Input: part model. Units: mm. Frame: model coordinates. A direction names the side the tool comes from. Round coordinates to 2 decimals unless told otherwise and drop trailing zeros. Loops run counter-clockwise (first coordinate to the right, second up) from the corner with the lowest first, then second, coordinate; pieces in that order, holes last. Notation, with made-up numbers: (11.5, 44.25) - (55.5, 44.25) arc R16 ccw to (55.5, 53.25) - close; hole circle Ø11 at (62, -23.75). An arc over 180 degrees is marked (long way). Write each question's results on one line, items separated by ' | '.
from build123d import *

# Parameters (mm, degrees)
F1_DEPTH = 25
F2_R     = 0.8


# Not quite as in the source:
# - a feature names something its author has since deleted; it is built from what else it names


with BuildPart() as f1:
    # F0 (on Top) → F1 (new body)
    with BuildSketch(Plane.XY):
        Polygon((-15.2705168036, 4.776119403), (-17.6585765051, -2.8591389988), (-14.7953546044, -3.7546613869), (-13.302817291, 1.0173751143), (-3.7587442887, -1.9676995126), (-21.9676995126, -60.1865448263), (-31.5117725148, -57.2014701994), (-30.0192352014, -52.4294336983), (-32.8824571021, -51.5339113102), (-35.2705168036, -59.169169712), (-20, -63.945289115), (-19.0616978853, -60.945289115), (-0.4691510573, -1.5), (3.1308489427, -1.5), (3.1308489427, -10), (6.1308489427, -10), (6.1308489427, -4.0311980993), (6.1308489427, 0), (0, 0), align=None)
        Polygon((0, -60.945289115), (-19.0616978853, -60.945289115), (-20, -63.945289115), (0, -63.945289115), align=None)
        Polygon((9.5918557882, -1.385692507), (6.1308489427, 0), (6.1308489427, -4.0311980993), (9.5918557882, -2.7201510966), align=None)
    extrude(amount=F1_DEPTH)

    # F2
    f2_edges = [f1.edges().sort_by_distance(p)[0] for p in [
        (-15.270517, 4.776119, 12.5),
        (-17.658577, -2.859139, 12.5),
        (-14.795355, -3.754661, 12.5),
        (-32.882457, -51.533911, 12.5),
        (-35.270517, -59.16917, 12.5),
        (-30.019235, -52.429434, 12.5),
        (-20, -63.945289, 12.5),
        (6.130849, -10, 12.5),
        (3.130849, -10, 12.5),
        (0, -60.945289, 12.5),
        (0, -63.945289, 12.5),
        (9.591856, -1.385693, 12.5),
        (9.591856, -2.720151, 12.5),
        (0, 0, 12.5),
        (6.130849, 0, 12.5),
        (6.130849, -4.031198, 12.5),
    ]]
    fillet(f2_edges, radius=F2_R)


solid = f1.part
1. Section query A-A, the plane x = -1.5. Output: boundary loops of the cut face in (y, z).
Answer:
outline: (-63.95, 0) - (-60.95, 0) - (-60.95, 25) - (-63.95, 25) - close; (-4.8, 0) - (0.47, 0) - (0.47, 25) - (-4.8, 25) - close
2. Section query C-C, the plane y = -30.5. Output: boundary loops of the cut face in (x, z).
Answer:
outline: (-12.68, 0) - (-9.54, 0) - (-9.54, 25) - (-12.68, 25) - close
3. Section query B-B, the plane x = -10. Output: boundary loops of the cut face in (y, z), plus the area to 3 significant figures.
Answer:
outline: (-63.95, 0) - (-60.95, 0) - (-60.95, 25) - (-63.95, 25) - close; (-31.97, 0) - (-21.92, 0) - (-21.92, 25) - (-31.97, 25) - close; (-0.02, 0) - (3.13, 0) - (3.13, 25) - (-0.02, 25) - close | area: 405 mm^2
4. Contact query for flat-ended pins moving along their axis: pin 1 (8 mm diameter, centred on x = 4.5, z = 20, fed in from +Y); pin 2 (10 mm diameter, centred on y = -12.5, z = 7.5, fed in from -X); pin 3 (1.4 mm diameter, centred on y = -7.5, z = 14, fed in from +X). Output: stop coordinate, or through.
Answer:
pin 1: y = 0 | pin 2: x = -8.62 | pin 3: x = 6.13
5. Mould query, pull axis Y, two halves, no side actions, for faces 1 (the flat face through (-7.211, 2.255, 12.325)), 2 (the flat face through (-9.896, -31.639, 12.325)), 3 (the flat face through (-10, -63.945, 12)). Classes: pulls with the +Y half, pulls with the -Y half, needs draft (parallel to the pull), parting line crosses it, or undercut.
Answer:
face 1: pulls with the +Y half | face 2: undercut | face 3: pulls with the -Y half
6. Section query D-D, the plane x = -29.5. Output: boundary loops of the cut face in (y, z).
Answer:
outline: (-60.97, 0) - (-57.83, 0) - (-57.83, 25) - (-60.97, 25) - close
7. Line query: line 1 (Y direction, x = 1.5, z = 16.5); line 2 (X direction, y = -2.5, z = 22); line 3 (X direction, y = -54, z = 16). Output: solid intervals per line, ascending. Write a range as [from, to].
Answer:
line 1: [-1.5, 0] | line 2: [-17.44, -14.4], [-3.93, -0.78], [3.13, 9.52] | line 3: [-33.65, -30.51], [-20.03, -16.89]
8. Set-up query: faces 4 (the flat face through (-31.441, -51.985, 12.325)), 5 (the flat face through (-13.938, -1.015, 12.325)), 6 (the flat face through (5, -10, 12)), 7 (the flat face through (3.131, -5, 12)). Return all of +Z, -Z, +X, -X, +Y, -Y with unobstructed straight access to the full face (end or side cutting, diameter ignored); none if empty.
Answer:
face 4: +Z, -Z, +Y | face 5: +Z, -Z | face 6: +Z, -Z, +X, -Y | face 7: +Z, -Z, -Y
